```python
from build123d import *

# Parameters (mm, degrees)
F0_R      = 2.5
F1_DEPTH  = 36
F4_DEPTH  = 3
F6_R      = 3.5
F7_DEPTH  = 1
F9_R      = 3.5
F10_DEPTH = 1
F13_DEPTH = 3
F16_DEPTH = 3
F18_R     = 1
F19_DEPTH = 69.001
F17_R     = 1
F20_DEPTH = 59.001


with BuildPart() as f1:
    # F0 (on Right) → F1 (new body, symmetric)
    with BuildSketch(Plane.YZ):
        Circle(F0_R)
    extrude(amount=F1_DEPTH, both=True)

    # F3 (on offset) → F4 (join)
    with BuildSketch(Plane.YZ.offset(-32)):
        Polygon((3.7, -1.75), (3.7, 1.75), (1, 3.75), (-11, 2.25), (-11, -2.25), (1, -3.75), align=None)
    extrude(amount=F4_DEPTH)

    # F6 (on offset) → F7 (join)
    with BuildSketch(Plane.YZ.offset(-13)):
        Circle(F6_R)
    extrude(amount=F7_DEPTH)

    # F9 (on offset) → F10 (join)
    with BuildSketch(Plane.YZ.offset(3)):
        Circle(F9_R)
    extrude(amount=F10_DEPTH)

    # F12 (on offset) → F13 (join)
    with BuildSketch(Plane.YZ.offset(33)):
        Polygon((-1, 3.75), (-3.7, 1.75), (-3.7, -1.75), (-1, -3.75), (11, -2.25), (11, 2.25), align=None)
    extrude(amount=-F13_DEPTH)

    # F15 (on offset) → F16 (join)
    with BuildSketch(Plane.YZ.offset(23)):
        Polygon((3.7, -1.75), (3.7, 1.75), (1, 3.75), (-11, 2.25), (-11, -2.25), (1, -3.75), align=None)
    extrude(amount=-F16_DEPTH)

    # F18 (on face) → F19 (cut, through all)
    with BuildSketch(Plane.YZ.offset(33)):
        with Locations((8, 0)):
            Circle(F18_R)
    extrude(amount=-F19_DEPTH, mode=Mode.SUBTRACT)

    # F17 (on face) → F20 (cut, through all)
    with BuildSketch(Plane.YZ.offset(23)):
        with Locations((-8, 0)):
            Circle(F17_R)
    extrude(amount=-F20_DEPTH, mode=Mode.SUBTRACT)


solid = f1.part
```
Verification items for the finished model (mm, model axes). A direction names the side the tool comes from. Coordinates: 2 decimals unless noted, no trailing zeros. Loops run counter-clockwise (first coordinate to the right, second up) from the corner with the lowest first, then second, coordinate; pieces in that order, holes last. Notation, with made-up numbers: (45, 22.5) -> (95, 22.5) arc R29 ccw to (95, 59.5) -> close; hole circle Ø5 at (-7.5, 18). An arc over 180 degrees is marked (long way). Answer in a Markdown table with one row per item.
1) Scan lines: line 1 along X through (y, z) = (-3.25, 1); line 2 along X through (y, z) = (-5.5, -0.5); line 3 along X through (y, z) = (8, -2.5). Record each from-to range of solid material in increasing order. Write a range as from..to.
The answers:
| item | result |
|---|---|
| line 1 | x = -32..-29, -13..-12, 3..4, 20..23, 30..33 |
| line 2 | x = -32..-29, 20..23 |
| line 3 | x = 30..33 |
2) Access from +Z, -Z, +X, -X, +Y, -Y to the whole of each face (thin tool, end or side, straight path). Record for faces 1 (the face through (34.52, -0.54, -2.44)), 2 (the face through (21.521, 2.369, 2.736)), 3 (the face through (-12, 2, -2)), 4 (the face through (32, -3.7, 0)).
The answers:
| item | result |
|---|---|
| face 1 | +X |
| face 2 | +Z, -X, +Y |
| face 3 | none |
| face 4 | +Z, -Z, +X, -Y |
3) Section check B-B (y = -8). Record the cut outline in (x, z) (3 decimals), and give its area (3 significant figures).
The answers:
| item | result |
|---|---|
| outline | (-32, -2.625) -> (-29, -2.625) -> (-29, -1) -> (-32, -1) -> close; (-32, 1) -> (-29, 1) -> (-29, 2.625) -> (-32, 2.625) -> close; (20, -2.625) -> (23, -2.625) -> (23, -1) -> (20, -1) -> close; (20, 1) -> (23, 1) -> (23, 2.625) -> (20, 2.625) -> close |
| area | 19.5 mm2 |
4) Depth check by flat-ended pin: P1, Ø5, axis at x = -12, y = 2, coming from the +Z side; P2, Ø1, axis at x = 23, y = 2, coming from the +Z side; P3, Ø4, axis at x = 10, z = 0.5, coming from the +Y side; P4, Ø1.6, axis at y = -8, z = 0, coming from the +X side. Enter the tip coordinate at first touch or a pass-through.
The answers:
| item | result |
|---|---|
| P1 | stops at z = 3.5 |
| P2 | stops at z = 3.38 |
| P3 | stops at y = 2.5 |
| P4 | passes through |
5) Section check C-C (z = 0). Give the number of separate pieces and of enclosed holes in the cut face, and give its area (3 significant figures).
The answers:
| item | result |
|---|---|
| separate pieces | 4 |
| enclosed holes | 0 |
| area | 433 mm2 |
6) Section check A-A (x = -30). Record the cut outline in (y, z).
The answers:
| item | result |
|---|---|
| outline | (-11, -2.25) -> (1, -3.75) -> (3.7, -1.75) -> (3.7, 1.75) -> (1, 3.75) -> (-11, 2.25) -> close; hole circle Ø2 at (-8, 0) |
7) Section check D-D (y = 5.5). Record the cut outline in (x, z), and give its area (3 significant figures).
The answers:
| item | result |
|---|---|
| outline | (30, -2.94) -> (33, -2.94) -> (33, 2.94) -> (30, 2.94) -> close |
| area | 17.6 mm2 |
8) Draft check along X on faces 5 (the face through (36, 0, 0)), 6 (the face through (4, 2, -2)), 7 (the face through (-20.89, -0.54, -2.44)), 8 (the face through (22, -11, 0)). Enter one of: released by +X, released by -X, zero draft, split by the parting line, or undercut.
The answers:
| item | result |
|---|---|
| face 5 | released by +X |
| face 6 | undercut |
| face 7 | undercut |
| face 8 | zero draft |
